from build123d import *

# Parameters (mm, degrees)
CYLINDER051_R     = 3
CYLINDER051_DEPTH = 18
CYLINDER050_R     = 3
CYLINDER050_DEPTH = 51


with BuildPart() as cylindre047:
    # Cylinder051 → Cylinder051 (new body)
    with BuildSketch(Plane(origin=(-32, 9, -130), x_dir=(1, 0, 0), z_dir=(0, 0, 1))):
        Circle(CYLINDER051_R)
    extrude(amount=CYLINDER051_DEPTH)


with BuildPart() as fusion025:
    # Cylinder050 → Cylinder050 (new body)
    with BuildSketch(Plane(origin=(-32, 9, -128), x_dir=(0, 0, -1), z_dir=(1, 0, 0))):
        Circle(CYLINDER050_R)
    extrude(amount=CYLINDER050_DEPTH)

    # Fusion025: union Cylindre047
    add(cylindre047.part)


solid = fusion025.part
CAD build for the part. Positions are in the model's coordinates, mm. A direction names the side the tool comes from. Give positions to 0.01 mm unless a question says otherwise; leave off trailing zeros. Order: outer loops, then holes, each group sorted by start corner. A loop starts at its lowest first (then second) coordinate and runs counter-clockwise, first axis right, second up. Notation, with made-up numbers: (60, -21.5) - (80, -21.5) arc R30 ccw to (80, 0.5) - close; hole circle Ø4 at (-35, -0.5). An arc over 180 degrees is marked (long way). Write each question's results on one line, items separated by ' | '.
1. Probe L1, parallel to X at y = 9.1, z = -119.5; L2, parallel to Y at x = -19, z = -130; L3, parallel to Z at x = -2.5, y = 9.2. List the from-to ranges inside material, lowest first. Write a range as from..to.
Calculated:
L1: x = -35..-29 | L2: y = 6.76..11.24 | L3: z = -130.99..-125.01
2. Saw through at A-A on y = 9. List the corners of the cut face in (x, z), and give its area (3 significant figures).
Calculated:
outline: (-35, -130) - (-32, -130) - (-32, -131) - (19, -131) - (19, -125) - (-29, -125) - (-29, -112) - (-35, -112) - close | area: 399 mm2
3. Pin check, flat tips, straight feed: pin 1 (1 mm diameter, centred on x = -19.5, y = 7, fed in from +Z); pin 2 (1.5 mm diameter, centred on x = 8, y = 7, fed in from +Z); pin 3 (3 mm diameter, centred on x = -11.5, y = 9, fed in from +Z); pin 4 (2.5 mm diameter, centred on x = -32.5, y = 8.5, fed in from -Z). Stop position of each tip, or through.
Calculated:
pin 1: stops at z = -125.4 | pin 2: stops at z = -125.27 | pin 3: stops at z = -125 | pin 4: stops at z = -131
4. Saw through at C-C on x = -15.5. List the corners of the cut face in (y, z), and give its area (3 significant figures).
Calculated:
outline: circle Ø6 at (9, -128) | area: 28.3 mm2
5. Saw through at D-D on z = -128.5. List the corners of the cut face in (x, y).
Calculated:
outline: (-31.5, 6.04) - (19, 6.04) - (19, 11.96) - (-31.5, 11.96) arc R3 ccw (long way) to start
6. 3-axis set-ups, long thin cutter, end or side, ignore diameter. For faces 1 (the face through (-32, 9, -130.4)), 2 (the face through (-6.86, 9.9, -130.86)), 3 (the face through (19, 9, -128)): which of +Z, -Z, +X, -X, +Y, -Y reach the whole face in a straight line?
Calculated:
face 1: -Z, -X, +Y, -Y | face 2: +X | face 3: +Z, -Z, +X, +Y, -Y
7. Saw through at B-B on z = -120. List the corners of the cut face in (x, y).
Calculated:
outline: circle Ø6 at (-32, 9)
